from build123d import *

# Parameters (mm, degrees)
BOSS_EXTRUDE1_DEPTH = 190
FILLET1_R           = 2
SKETCH2_W           = 4
SKETCH2_H           = 3
BOSS_EXTRUDE2_DEPTH = 2
SKETCH3_W           = 4
SKETCH3_H           = 5
BOSS_EXTRUDE3_DEPTH = 3
CUT_EXTRUDE2_DEPTH  = 193.294695715
FILLET2_R           = 1
FILLET3_R           = 1


with BuildPart() as part:
    # Sketch1 → Boss-Extrude1 (new body)
    with BuildSketch(Plane(origin=(0, 0, 0), x_dir=(0, 0, -1), z_dir=(1, 0, 0))):
        Polygon((-22.5, 0), (22.5, 0), (27.5, -3), (27.5, -6), (-27.5, -6), (-27.5, -3), align=None)
    extrude(amount=BOSS_EXTRUDE1_DEPTH)

    # Fillet1
    fillet1_edges = [part.edges().sort_by_distance(p)[0] for p in [
        (95, 0, 22.5),
        (95, 0, -22.5),
        (95, -3, -27.5),
        (95, -3, 27.5),
    ]]
    fillet(fillet1_edges, radius=FILLET1_R)

    # Sketch2 → Boss-Extrude2 (add)
    with BuildSketch(Plane.XZ.offset(6)):
        with Locations((32, -21)):
            Rectangle(SKETCH2_W, SKETCH2_H)
        with Locations((32, 21)):
            Rectangle(SKETCH2_W, SKETCH2_H)
        with Locations((66, -21)):
            Rectangle(SKETCH2_W, SKETCH2_H)
        with Locations((66, 21)):
            Rectangle(SKETCH2_W, SKETCH2_H)
        with Locations((158, -21)):
            Rectangle(SKETCH2_W, SKETCH2_H)
        with Locations((124, -21)):
            Rectangle(SKETCH2_W, SKETCH2_H)
        with Locations((124, 21)):
            Rectangle(SKETCH2_W, SKETCH2_H)
        with Locations((158, 21)):
            Rectangle(SKETCH2_W, SKETCH2_H)
    extrude(amount=BOSS_EXTRUDE2_DEPTH)

    # Sketch3 → Boss-Extrude3 (add)
    with BuildSketch(Plane.XZ.offset(8)):
        with Locations((32, -22)):
            Rectangle(SKETCH3_W, SKETCH3_H)
        with Locations((32, 22)):
            Rectangle(SKETCH3_W, SKETCH3_H)
        with Locations((66, -22)):
            Rectangle(SKETCH3_W, SKETCH3_H)
        with Locations((66, 22)):
            Rectangle(SKETCH3_W, SKETCH3_H)
        with Locations((158, -22)):
            Rectangle(SKETCH3_W, SKETCH3_H)
        with Locations((124, -22)):
            Rectangle(SKETCH3_W, SKETCH3_H)
        with Locations((124, 22)):
            Rectangle(SKETCH3_W, SKETCH3_H)
        with Locations((158, 22)):
            Rectangle(SKETCH3_W, SKETCH3_H)
    extrude(amount=BOSS_EXTRUDE3_DEPTH)

    # Sketch4 → Cut-Extrude2 (cut, through all)
    with BuildSketch(Plane.ZY):
        Polygon((-24.5, -8), (-21.3, -11), (-24.5, -11), align=None)
        Polygon((24.5, -8), (21.3, -11), (24.5, -11), align=None)
    extrude(amount=-CUT_EXTRUDE2_DEPTH, mode=Mode.SUBTRACT)

    # Fillet2
    fillet2_edges = [part.edges().sort_by_distance(p)[0] for p in [
        (32, -11, -19.5),
        (32, -11, 19.5),
        (66, -11, -19.5),
        (66, -11, 19.5),
        (158, -11, -19.5),
        (124, -11, -19.5),
        (124, -11, 19.5),
        (158, -11, 19.5),
    ]]
    fillet(fillet2_edges, radius=FILLET2_R)

    # Fillet3
    fillet3_edges = [part.edges().sort_by_distance(p)[0] for p in [
        (124, -6, -19.5),
        (122, -6, -21),
        (126, -6, -21),
        (122, -6, 21),
        (124, -6, 19.5),
        (126, -6, 21),
        (158, -6, 19.5),
        (160, -6, 21),
        (156, -6, 21),
        (30, -6, -21),
        (34, -6, -21),
        (32, -6, -19.5),
        (30, -6, 21),
        (32, -6, 19.5),
        (34, -6, 21),
        (68, -6, -21),
        (66, -6, -19.5),
        (64, -6, -21),
        (66, -6, 19.5),
        (68, -6, 21),
        (64, -6, 21),
        (160, -6, -21),
        (158, -6, -19.5),
        (156, -6, -21),
    ]]
    fillet(fillet3_edges, radius=FILLET3_R)


solid = part.part
CAD build for the part. Positions are in the model's coordinates, mm. A direction names the side the tool comes from. Coordinates: 2 decimals unless noted, no trailing zeros. Order: outer loops, then holes, each group sorted by start corner. A loop starts at its lowest first (then second) coordinate and runs counter-clockwise, first axis right, second up. Notation, with made-up numbers: (77, 89) -> (97, 89) arc R17 ccw to (97, 109) -> close; hole circle Ø9 at (39.25, 3). An arc over 180 degrees is marked (long way). Answer in a Markdown table with one row per item.
1) Drill centre lines: line 1 (Y direction, x = 28.5, z = 9); line 2 (Z direction, x = 155.5, y = -2.5); line 3 (Y direction, x = 89, z = -25). Where is each one in solid material? Low to high.
Check values:
| item | result |
|---|---|
| line 1 | -6 to 0 |
| line 2 | -26.66 to 26.66 |
| line 3 | -6 to -1.5 |
2) Band-saw the part on B-B (z = -11). List the corners of the cut face in (x, y).
Check values:
| item | result |
|---|---|
| outline | (0, -6) -> (190, -6) -> (190, 0) -> (0, 0) -> close |
3) Mould opens along X. For faces 1 (the face through (158, -9.5, -22.9)), 2 (the face through (122, -9, 21)), 3 (the face through (190, -3, 0)) say: pulls with the +X half, pulls with the -X half, needs draft (parallel to the pull), parting line crosses it, or undercut.
Check values:
| item | result |
|---|---|
| face 1 | needs draft |
| face 2 | undercut |
| face 3 | pulls with the +X half |
4) Flat gauge pins, fed straight in: P1, Ø3, axis at y = -9, z = -22, coming from the +X side; P2, Ø2, axis at y = -9.5, z = 22.5, coming from the -X side; P3, Ø2, axis at x = 32, z = -23.5, coming from the +Y side; P4, Ø5, axis at x = 34.5, z = 20.5, coming from the -Y side. Where does each tip first touch, or does it go through?
Check values:
| item | result |
|---|---|
| P1 | x = 160 |
| P2 | x = 30 |
| P3 | y = -0.08 |
| P4 | y = -11 |
5) Band-saw the part on C-C (x = 124). List the corners of the cut face in (y, z).
Check values:
| item | result |
|---|---|
| outline | (-11, -21.3) -> (-8, -24.5) -> (-8, -22.5) -> (-6, -22.5) -> (-6, -27.5) -> (-4.13, -27.5) arc R2 ccw to (-2.42, -26.53) -> (-0.29, -22.98) arc R2 ccw to (0, -21.95) -> (0, 21.95) arc R2 ccw to (-0.29, 22.98) -> (-2.42, 26.53) arc R2 ccw to (-4.13, 27.5) -> (-6, 27.5) -> (-6, 22.5) -> (-8, 22.5) -> (-8, 24.5) -> (-11, 21.3) -> (-11, 20.5) arc R1 ccw to (-10, 19.5) -> (-7, 19.5) arc R1 cw to (-6, 18.5) -> (-6, -18.5) arc R1 cw to (-7, -19.5) -> (-10, -19.5) arc R1 ccw to (-11, -20.5) -> close |
6) Which spindle directions (+Z, -Z, +X, -X, +Y, -Y) get a long thin tool onto all of the face, cutting with end or side? Do faces 4 (the face through (32, -8, 19.5)), 5 (the face through (160, -9, -21)), 6 (the face through (68, -9, -21)), 7 (the face through (30, -9, 21)), 8 (the face through (93.67, -1.37, 24.78)). Say none if no direction does.
Check values:
| item | result |
|---|---|
| face 4 | +X, -X, -Y |
| face 5 | +Z, -Z, +X, -Y |
| face 6 | +Z, -Z, -Y |
| face 7 | +Z, -Z, -X, -Y |
| face 8 | +Z, +X, -X, +Y |
7) Band-saw the part on A-A (x = 95.5). List the corners of the cut face in (y, z).
Check values:
| item | result |
|---|---|
| outline | (-6, -27.5) -> (-4.13, -27.5) arc R2 ccw to (-2.42, -26.53) -> (-0.29, -22.98) arc R2 ccw to (0, -21.95) -> (0, 21.95) arc R2 ccw to (-0.29, 22.98) -> (-2.42, 26.53) arc R2 ccw to (-4.13, 27.5) -> (-6, 27.5) -> close |
